The listing builds one solid part. Answer for the finished solid, in the listing's coordinates (mm). Give positions to 0.01 mm unless a question says otherwise; leave off trailing zeros. Order: outer loops, then holes, each group sorted by start corner. A loop starts at its lowest first (then second) coordinate and runs counter-clockwise, first axis right, second up. Notation, with made-up numbers: (-35, 18.5) - (21, 18.5) arc R11 cw to (21, 23.5) - close; hole circle Ø2 at (2.25, 20). An arc over 180 degrees is marked (long way). Use CSV: the item, a comma, the result in double quotes.
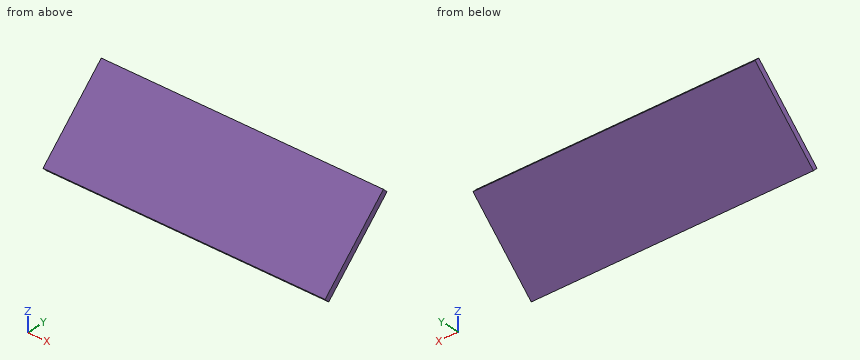
```python
from build123d import *

# Parameters (mm, degrees)
F1_W     = 152.4
F1_H     = 50.8
F2_DEPTH = 3.175
F4_D     = 1.778
F4_DEPTH = 12.2464285714
F4_TIP   = 0.5341650903


with BuildPart() as f2:
    # F1 (on face) → F2 (new body)
    with BuildSketch(Plane(origin=(0, 0, 0), x_dir=(1, 0, 0), z_dir=(0, -0.7071067812, 0.7071067812))):
        with Locations((0, 25.4)):
            Rectangle(F1_W, F1_H)
    extrude(amount=F2_DEPTH)

    # F4
    with Locations(Plane.YZ.offset(76.2)):
        with Locations((3.3675965891, 5.6126595319)):
            Hole(F4_D / 2, depth=F4_DEPTH)
            with Locations((0, 0, -(F4_DEPTH + F4_TIP / 2))):  # 118° drill point
                Cone(0, F4_D / 2, F4_TIP, mode=Mode.SUBTRACT)

    # F5: F2 across plane


with BuildPart() as f2_1:
    add(f2.part)
    add(f2.part.mirror(Plane.YZ))


solid = f2_1.part
```
Item 1: The part is cut by section B-B (y = 27.5). Give the vertices of the cut face in (x, z).
Taken from the geometry:
outline,"(-76.2, 27.5) - (76.2, 27.5) - (76.2, 31.99) - (-76.2, 31.99) - close"
Item 2: Each of these flat-tipped pins is pushed along its axis until it touches: pin 1 (2 mm diameter, centred on x = 56, y = 24.5, fed in from -Z); pin 2 (5 mm diameter, centred on x = 42, z = 10, fed in from +Y); pin 3 (6 mm diameter, centred on x = -36, y = 28, fed in from +Z); pin 4 (10 mm diameter, centred on y = 8, z = 25, fed in from +X). Where does it stop, or does it pass through?
Taken from the geometry:
pin 1,"z = 23.5"
pin 2,"y = 12.5"
pin 3,"z = 35.49"
pin 4,"through"
Item 3: Find the intervals of material crossed by line 1 along Y through (x, z) = (51, 9); line 2 along Z through (x, y) = (64.5, 18.5); line 3 along Z through (x, y) = (-63, 8), in increasing order.
Taken from the geometry:
line 1,"4.51 to 9"
line 2,"18.5 to 22.99"
line 3,"8 to 12.49"
Item 4: The part is cut by section A-A (x = 36.5). Give the vertices of the cut face in (y, z).
Taken from the geometry:
outline,"(-2.25, 2.25) - (0, 0) - (35.92, 35.92) - (33.68, 38.17) - close"
